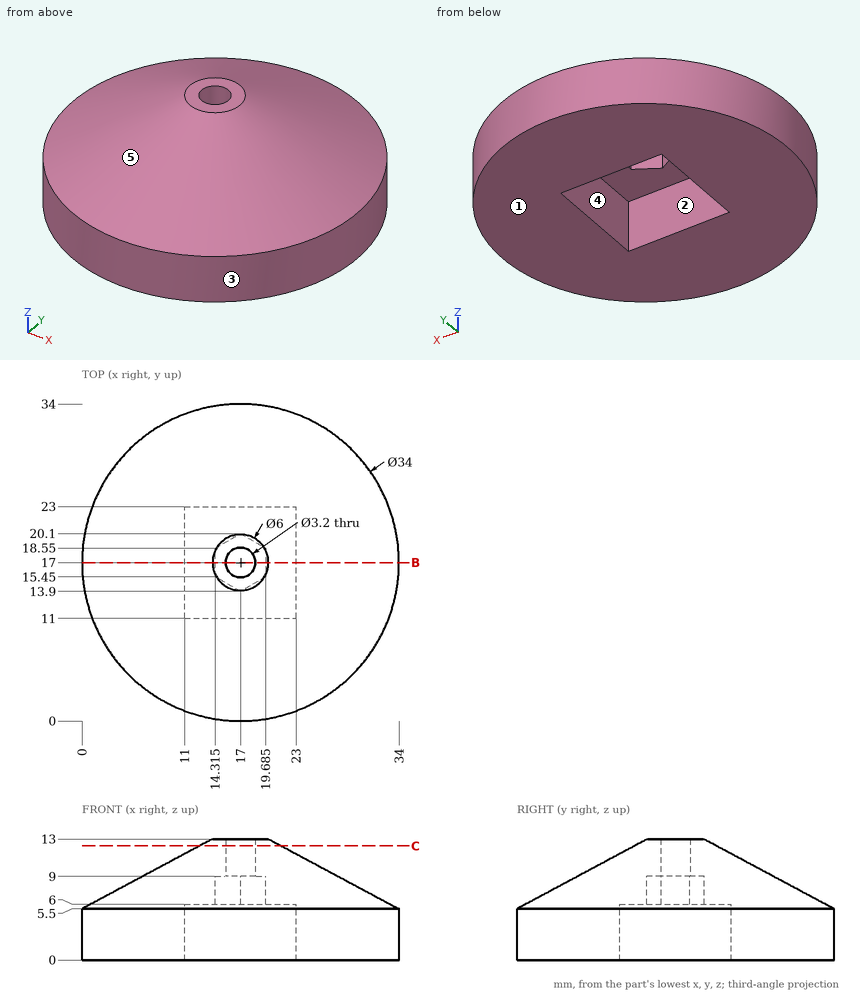
Input: dimensioned drawing with shaded views. Units: mm. Origin: part minimum x, y, z. A direction names the side the tool comes from. Give positions to 0.01 mm unless a question says otherwise; leave off trailing zeros. Order: outer loops, then holes, each group sorted by start corner. A loop starts at its lowest first (then second) coordinate and runs counter-clockwise, first axis right, second up. Notation, with made-up numbers: (25.25, 82) -> (52.25, 82) arc R27 ccw to (52.25, 118) -> close; hole circle Ø11 at (-21.5, 29). An arc over 180 degrees is marked (long way). Use a Markdown table: item, result.
1) Mould query, pull axis X, two halves, no side actions, for the marked faces 1, 2 and 3. Classes: +X half, -X half, draft (parallel to the pull), parting line (faces both ways), or undercut.
Answer list:
| item | result |
|---|---|
| face 1 | draft |
| face 2 | undercut |
| face 3 | parting line |
2) Contact query for flat-ended pins moving along their axis: P1, Ø3.5, axis at y = 17, z = 7, coming from the -X side; P2, Ø1.8, axis at x = 19.5, z = 2, coming from the +Y side; P3, Ø6, axis at x = 14.5, y = 17, coming from the -Z side; P4, Ø1.6, axis at x = 16.5, y = 17.5, coming from the -Z side. Output: stop coordinate, or through.
Answer list:
| item | result |
|---|---|
| P1 | x = 0 |
| P2 | y = 33.92 |
| P3 | z = 6 |
| P4 | through |
3) Ray query, line 1 along X through (y, z) = (17, 12.05) (1 decimal); line 2 along X through (y, z) = (17, 10.2) (1 decimal); line 3 along Y through (x, z) = (17, 12.1). Return the intervals inside material, ascending. Write a range as [from, to].
Answer list:
| item | result |
|---|---|
| line 1 | [12.2, 15.4], [18.6, 21.8] |
| line 2 | [8.8, 15.4], [18.6, 25.2] |
| line 3 | [12.32, 15.4], [18.6, 21.68] |
4) Section query C-C, the plane z = 12.25. Return the cut outline in (x, y).
Answer list:
| item | result |
|---|---|
| outline | circle Ø8.8 at (17, 17); hole circle Ø3.2 at (17, 17) |
5) Reachability of the marked faces 4 and 5 from +Z, -Z, +X, -X, +Y, -Y: full face, straight path, thin tool, end or side. Return the list, or none.
Answer list:
| item | result |
|---|---|
| face 4 | -Z |
| face 5 | +Z |
6) Section query B-B, the plane y = 17. Return the cut outline in (x, z) (1 decimal), then the cut area to 3 significant figures.
Answer list:
| item | result |
|---|---|
| outline | (0, 0) -> (11, 0) -> (11, 6) -> (14.3, 6) -> (14.3, 9) -> (15.4, 9) -> (15.4, 13) -> (14, 13) -> (0, 5.5) -> close; (18.6, 9) -> (19.7, 9) -> (19.7, 6) -> (23, 6) -> (23, 0) -> (34, 0) -> (34, 5.5) -> (20, 13) -> (18.6, 13) -> close |
| area | 236 mm² |
